The model under review builds one solid part; all positions refer to its coordinate system, in mm. A direction names the side the tool comes from. Give positions to 0.01 mm unless a question says otherwise; leave off trailing zeros. Loops run counter-clockwise (first coordinate to the right, second up) from the corner with the lowest first, then second, coordinate; pieces in that order, holes last. Notation, with made-up numbers: M -29.75,-30.75 L -24.75,-30.75 A34 cw -24.75,0.25 Z; hole C 28.5,60.25 d8. An arc over 180 degrees is marked long. Write item = value, one per line. Start each with the question number.
1. We need section C-C on z = -1.5. Give the boundary of the cut face in (x, y), then the cut area to 3 significant figures.
2. Wall thickness on line 1 along Z through (x, y) = (-0.5, -585); line 2 along X through (y, z) = (-956, 21.5): over which ranges is each line inside the solid? List them lowest first. Write a range as from..to.
3. Draft analysis for pull direction Z (two halves, no side actions). For faces 1 (the face through (25, -493, 0)), 2 (the face through (0, -493, 22)), 3 (the face through (0, -493, -25)), 4 (the face through (0, -493, 25)), state which applies: pulls with the +Z half, pulls with the -Z half, needs draft (parallel to the pull), parting line crosses it, or undercut.
4. We need section A-A on x = -6.5. Give the boundary of the cut face in (y, z), then the cut area to 3 significant figures.
5. For faces 5 (the face through (-22, -494, 0)), 6 (the face through (-0.1, -25.1, -22.3)), list the 3-axis set-ups (+Z, -Z, +X, -X, +Y, -Y) from which the entire face can be reached by the end or side of a thin tool; tool diameter is ignored.
6. We need section B-B on y = -514. Give the boundary of the cut face in (x, z).
from build123d import *

# Parameters (mm, degrees)
F0_W        = 50
F0_H        = 50
F0_W_2      = 44
F0_H_2      = 44
F1_DEPTH    = 1000
F2_T1_DEPTH = 307.1682987966


# Not quite as in the source:
# - a fillet or chamfer that OpenCascade refuses, or shapes differently, is made with other operations: its cross-section is extruded or revolved along the edge and cut away or added


with BuildPart() as f1:
    # F0 (on Front) → F1 (new body)
    with BuildSketch(Plane.XZ):
        Rectangle(F0_W, F0_H)
        Rectangle(F0_W_2, F0_H_2, mode=Mode.SUBTRACT)
    extrude(amount=F1_DEPTH)

    # F2: chamfer of 50 on 2 edges, made by hand

    # F2_s2 → F2_t1 (cut)
    with BuildSketch(Plane.XY.offset(-153.5841493983)):
        Polygon((-25, -950), (25, -1000), (-25, -1000), align=None)
        Polygon((-25, -50), (25, 0), (-25, 0), align=None)
    extrude(amount=F2_T1_DEPTH, mode=Mode.SUBTRACT)


solid = f1.part
Final values:
q1.outline = M -25,-950 L -22,-953 L -22,-47 L -25,-50 Z; M 22,-997 L 25,-1000 L 25,0 L 22,-3 Z
q1.area = 5,700 mm²
q2.line_1 = -25..-22, 22..25
q2.line_2 = 22..25
q3.face_1 = needs draft
q3.face_2 = undercut
q3.face_3 = pulls with the -Z half
q3.face_4 = pulls with the +Z half
q4.outline = M -968.5,-25 L -31.5,-25 L -31.5,-22 L -968.5,-22 Z; M -968.5,22 L -31.5,22 L -31.5,25 L -968.5,25 Z
q4.area = 5,620 mm²
q5.face_5 = +Y, -Y
q5.face_6 = +Z, -Z, -X, +Y
q6.outline = M -25,-25 L 25,-25 L 25,25 L -25,25 Z; hole M -22,-22 L 22,-22 L 22,22 L -22,22 Z
